Study the drawing (mm; zero at the part's minimum x, y, z) and answer. Coordinates: 2 decimals unless noted, no trailing zeros. Order: outer loops, then holes, each group sorted by start corner. A loop starts at its lowest first (then second) coordinate and runs counter-clockwise, first axis right, second up. Notation, with made-up numbers: M -17.5,20.25 L -6.5,20.25 A36 ccw -6.5,57.25 Z; hole C 65.5,71.5 d2. An arc over 180 degrees is marked long. Put each result on its own line as item: value.
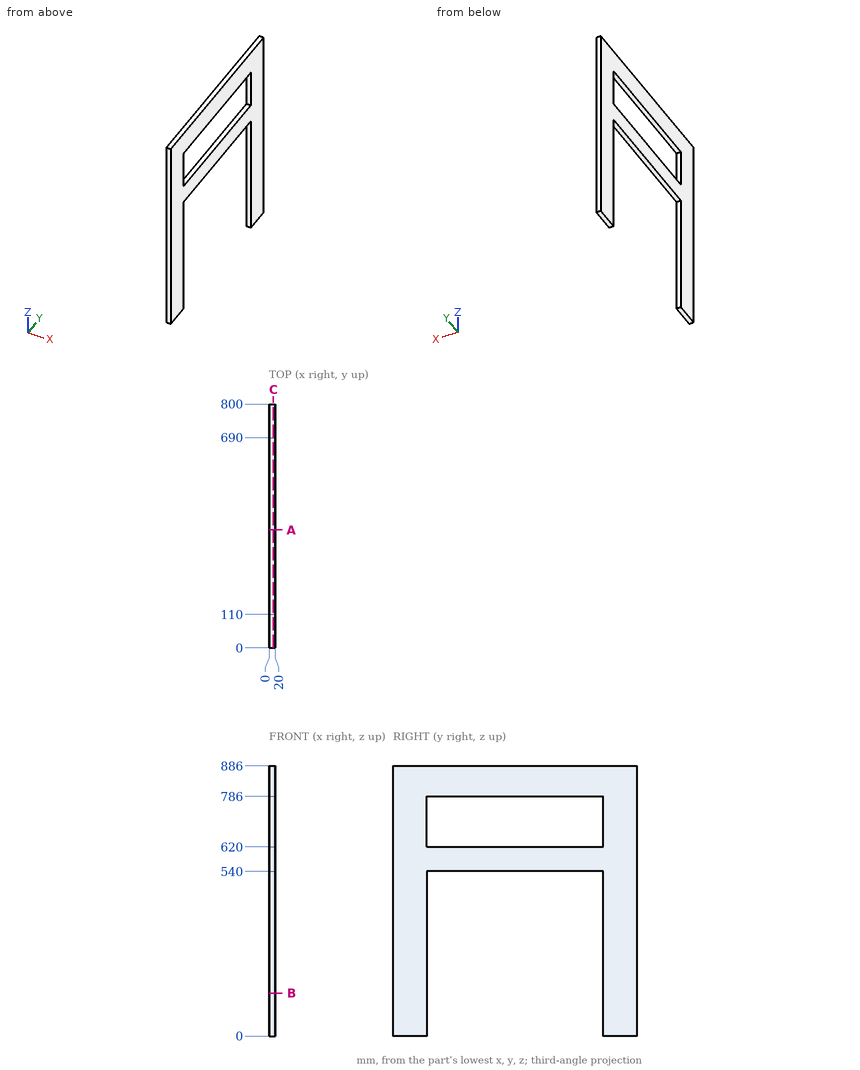
Q1. Find section A-A on y = 387. Write down the section's boundary in (x, z), plus the area to 3 significant figures.
Answers below:
outline: M 0,540 L 20,540 L 20,620 L 0,620 Z; M 0,786 L 20,786 L 20,886 L 0,886 Z
area: 3,600 mm^2
Q2. Consider line 1 along Y through (x, z) = (17.5, 781); line 2 along Z through (x, y) = (1, 167). Determine where each line is inside the solid, lowest interval first.
Answers below:
line 1: y = 0 to 110, 690 to 800
line 2: z = 540 to 620, 786 to 886
Q3. Given pin 1 (10 mm diameter, centred on x = 12, y = 366, fed in from -Z), flat-ended and moving along its own axis, determine where the tip first touches the part or whether it passes through.
Answers below:
pin 1: stops at z = 540
Q4. Find section B-B on z = 141. Write down the section's boundary in (x, y), plus the area to 3 significant figures.
Answers below:
outline: M 0,0 L 20,0 L 20,110 L 0,110 Z; M 0,690 L 20,690 L 20,800 L 0,800 Z
area: 4,400 mm^2
Q5. Find section C-C on x = 14.5. Write down the section's boundary in (y, z), plus the area to 3 significant figures.
Answers below:
outline: M 0,0 L 110,0 L 110,540 L 690,540 L 690,0 L 800,0 L 800,886 L 0,886 Z; hole M 110,620 L 690,620 L 690,786 L 110,786 Z
area: 299,000 mm^2
